```python
from build123d import *

# Parameters (mm, degrees)
F0_W     = 28.575
F0_H     = 31.75
F1_DEPTH = 1.5875
F3_DEPTH = 3.175
F4_W     = 38.1
F4_H     = 127
F4_W_2   = 3.175
F5_DEPTH = 3.175
F6_R     = 4
F6_R_2   = 1.85
F7_DEPTH = 25.4
F8_W     = 1.5875
F8_H     = 31.75
F9_DEPTH = 25.4


with BuildPart() as f1:
    # F0 (on Front) → F1 (new body)
    with BuildSketch(Plane.XZ):
        with Locations((-18.3960961165, 7.6425911009)):
            Rectangle(F0_W, F0_H)
    extrude(amount=F1_DEPTH)

    # F2 (on face) → F3 (join)
    with BuildSketch(Plane.YZ.offset(-4.1085961165)):
        Polygon((-38.1, -52.6824088991), (0, -52.6824088991), (0, -8.2324088991), (-1.5875, -8.2324088991), (-1.5875, 23.5175911009), (0, 23.5175911009), (0, 74.3175911009), (-38.1, 74.3175911009), align=None)
    extrude(amount=-F3_DEPTH)

    # F4 (on face) → F5 (join)
    with BuildSketch(Plane.XZ.offset(38.1)):
        with Locations((14.9414038835, 10.8175911009)):
            Rectangle(F4_W, F4_H)
        with Locations((-5.6960961165, 10.8175911009)):
            Rectangle(F4_W_2, F4_H)
    extrude(amount=F5_DEPTH)

    # F6 (on face) → F7 (cut)
    with BuildSketch(Plane.XZ.offset(1.5875)):
        with Locations((-16.6835961165, 7.6425911009)):
            Circle(F6_R)
        with Locations((-22.340450366, 13.2994453504)):
            Circle(F6_R_2)
        with Locations((-16.6835961165, 15.6425911009)):
            Circle(F6_R_2)
        with Locations((-11.026741867, 13.2994453504)):
            Circle(F6_R_2)
        with Locations((-11.026741867, 1.9857368514)):
            Circle(F6_R_2)
        with Locations((-16.6835961165, -0.3574088991)):
            Circle(F6_R_2)
        with Locations((-22.340450366, 1.9857368514)):
            Circle(F6_R_2)
        with Locations((-24.6835961165, 7.6425911009)):
            Circle(F6_R_2)
    extrude(amount=-F7_DEPTH, mode=Mode.SUBTRACT)

    # F8 (on face) → F9 (cut)
    with BuildSketch(Plane(origin=(-32.6835961165, 0, 0), x_dir=(0, -1, 0), z_dir=(-1, 0, 0))):
        with Locations((0.79375, 7.6425911009)):
            Rectangle(F8_W, F8_H)
    extrude(amount=-F9_DEPTH, mode=Mode.SUBTRACT)


solid = f1.part
```
Work out the finished part from the listing and answer in its coordinate system (mm). A direction names the side the tool comes from. Coordinates: 2 decimals unless noted, no trailing zeros. Write each loop counter-clockwise with the first axis right and the second up, starting at its lowest first coordinate (ties: lowest second). Pieces come first, ordered by that corner, then holes.
Q1. A cutting plane is placed at B-B, the plane x = 13. Give the vertices of the cut face in (y, z) (3 decimals), then the cut area to 3 significant figures.
Q2. A cutting plane is placed at C-C, the plane y = -27.5. Give the vertices of the cut face in (x, z).
Q3. Which of the six approach directions +Z, -Z, +X, -X, +Y, -Y give full straight-line access (tool end or side, diameter ignored) to faces 1 (the face through (15, -38.1, 12)), 2 (the face through (4, -39, 74.318))?
Q4. A cutting plane is placed at A-A, the plane z = -3. Give the vertices of the cut face in (x, y) (3 decimals).
Q5. Find the intervals of material crossed by line 1 (Y direction, x = 32.5, z = 28.5) (3 decimals); line 2 (X direction, y = -12, z = 46), in increasing order.
Q6. Each of these flat-tipped pins is pushed along its axis until it touches: pin 1 Ø10 at (x, y) = (14, -35.5) entering from -Z; pin 2 Ø1.5 at (y, z) = (-8, -2.5) entering from +X; pin 3 Ø12 at (x, z) = (5.5, -36.5) entering from +Y. Where does it stop, or does it pass through?
Findings below:
1. outline: (-41.275, -52.682) - (-38.1, -52.682) - (-38.1, 74.318) - (-41.275, 74.318) - close
1. area: 403 mm2
2. outline: (-7.28, -52.68) - (-4.11, -52.68) - (-4.11, 74.32) - (-7.28, 74.32) - close
3. face 1: +Z, -Z, +X, +Y
3. face 2: +Z, +X, -X, +Y, -Y
4. outline: (-7.284, -41.275) - (33.991, -41.275) - (33.991, -38.1) - (-4.109, -38.1) - (-4.109, 0) - (-7.284, 0) - close
5. line 1: y = -41.275 to -38.1
5. line 2: x = -7.28 to -4.11
6. pin 1: stops at z = -52.68
6. pin 2: stops at x = -4.11
6. pin 3: stops at y = -38.1
